Job drawing, mm, ordinate dimensions from the low corner. One solid piece. Coordinates: 2 decimals unless noted, no trailing zeros. Write each loop counter-clockwise with the first axis right and the second up, starting at its lowest first coordinate (ties: lowest second). Pieces come first, ordered by that corner, then holes. Notation, with made-up numbers: (22.5, 37) -> (57.5, 37) arc R24 cw to (57.5, 72) -> close; hole circle Ø11 at (13, 56). An arc over 180 degrees is marked (long way). One line per question, with ' | ' between items. Start each with the question number.
Item 1: Saw through at C-C (x = 10). List the corners of the cut face in (y, z), and give its area (3 significant figures).
Item 2: Pin check, flat tip, straight feed: pin 1 (5.5 mm diameter, centred on x = 60, z = 7, fed in from +Y). Stop position of the tip, or through.
Item 3: Probe probe 1 along X at (y, z) = (1, 30.5); probe 2 along X at (y, z) = (2.25, 96); probe 3 along Z at (x, y) = (59, 1.75). List the from-to ranges inside material, lowest first. Write a range as [from, to].
Item 4: Saw through at A-A (z = 79). List the corners of the cut face in (x, y), and give its area (3 significant figures).
Item 5: Saw through at B-B (y = 6.5). Count the separate pieces of the cut face and the enclosed holes in it, and give its area (3 significant figures).
Item 6: Saw through at D-D (z = 100). List the corners of the cut face in (x, y), and give its area (3 significant figures).
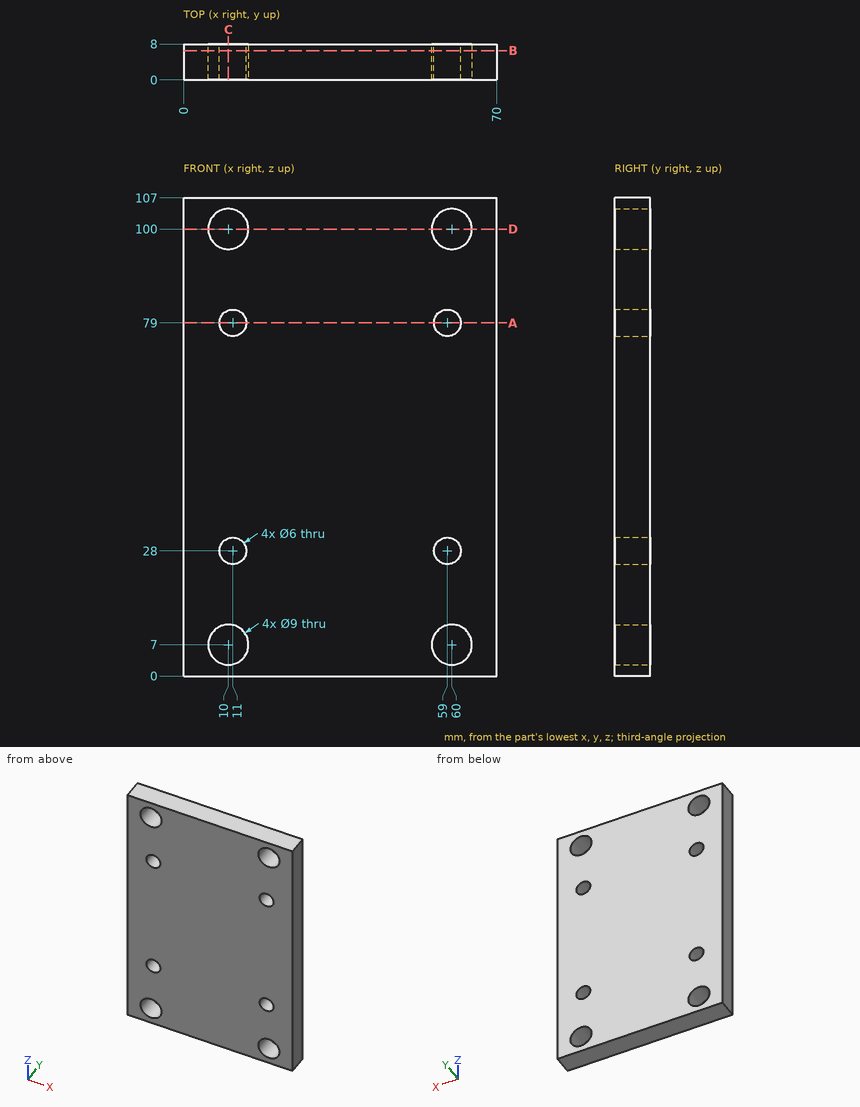
From the geometry:
1) outline: (0, 0) -> (8, 0) -> (8, 2.5) -> (0, 2.5) -> close; (0, 11.5) -> (8, 11.5) -> (8, 25.17) -> (0, 25.17) -> close; (0, 30.83) -> (8, 30.83) -> (8, 76.17) -> (0, 76.17) -> close; (0, 81.83) -> (8, 81.83) -> (8, 95.5) -> (0, 95.5) -> close; (0, 104.5) -> (8, 104.5) -> (8, 107) -> (0, 107) -> close | area: 621 mm2
2) pin 1: through
3) probe 1: [0, 9.34], [12.66, 57.34], [60.66, 70] | probe 2: [0, 7.94], [12.06, 57.94], [62.06, 70] | probe 3: [0, 2.61], [11.39, 25], [31, 76], [82, 95.61], [104.39, 107]
4) outline: (0, 0) -> (8, 0) -> (8, 8) -> (0, 8) -> close; (14, 0) -> (56, 0) -> (56, 8) -> (14, 8) -> close; (62, 0) -> (70, 0) -> (70, 8) -> (62, 8) -> close | area: 464 mm2
5) separate pieces: 1 | enclosed holes: 8 | area: 7,120 mm2
6) outline: (0, 0) -> (5.5, 0) -> (5.5, 8) -> (0, 8) -> close; (14.5, 0) -> (55.5, 0) -> (55.5, 8) -> (14.5, 8) -> close; (64.5, 0) -> (70, 0) -> (70, 8) -> (64.5, 8) -> close | area: 416 mm2
